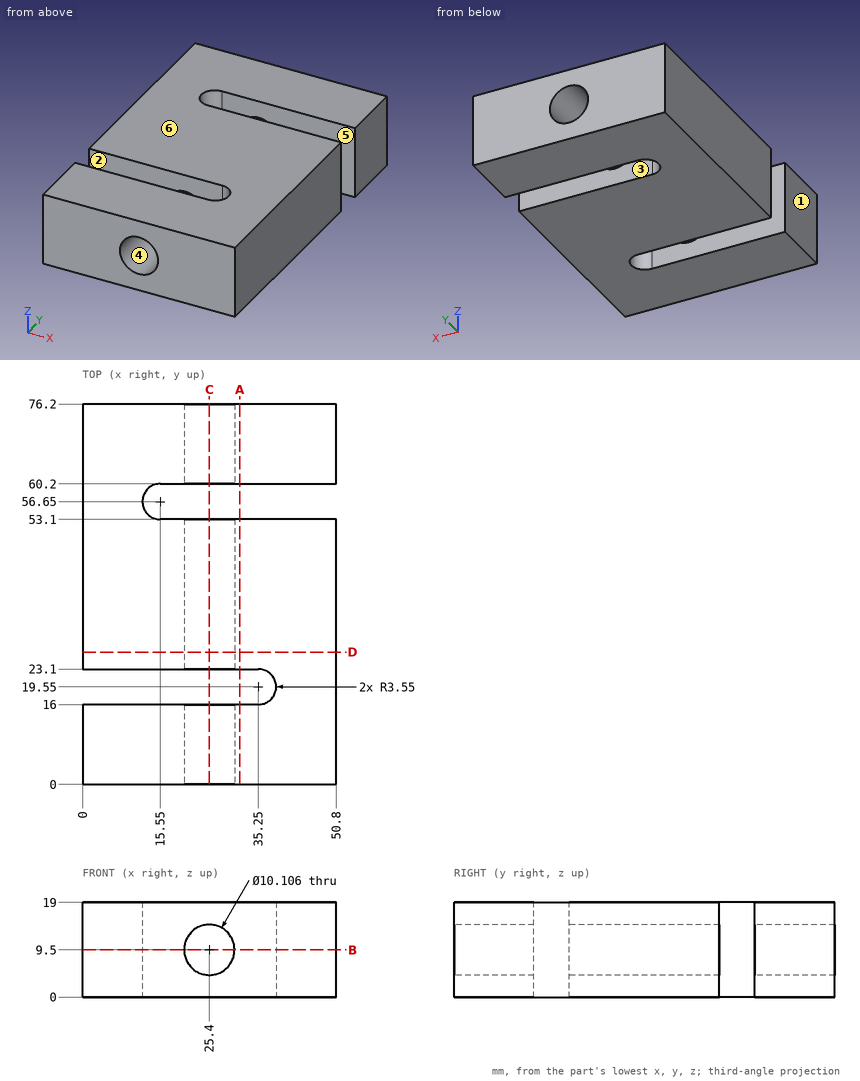
For this review, use the dimensioned drawing (mm, ordinates from the lowest corner) and the shaded views. A direction names the side the tool comes from. Round coordinates to 2 decimals unless told otherwise and drop trailing zeros. Loops run counter-clockwise (first coordinate to the right, second up) from the corner with the lowest first, then second, coordinate; pieces in that order, holes last. Notation, with made-up numbers: M -31.5,20.5 L -5.5,20.5 A25 cw -5.5,52.5 Z; hole C 51.25,-4.5 d9. An arc over 180 degrees is marked long. Answer as CSV lines item,"result".
1. We need section D-D (y = 26.5). Give the boundary of the cut face in (x, z), plus the area to 3 significant figures.
Outcome:
outline,"M 0,0 L 50.8,0 L 50.8,19 L 0,19 Z; hole C 25.4,9.5 d10.11"
area,"885 mm2"
2. We need section B-B (z = 9.5). Give the boundary of the cut face in (x, y).
Outcome:
outline,"M 0,0 L 20.35,0 L 20.35,16 L 0,16 Z; M 0,23.1 L 20.35,23.1 L 20.35,53.1 L 15.55,53.1 A3.55 cw 15.55,60.2 L 20.35,60.2 L 20.35,76.2 L 0,76.2 Z; M 30.45,0 L 50.8,0 L 50.8,53.1 L 30.45,53.1 L 30.45,23.1 L 35.25,23.1 A3.55 cw 35.25,16 L 30.45,16 Z; M 30.45,60.2 L 50.8,60.2 L 50.8,76.2 L 30.45,76.2 Z"
3. We need section A-A (x = 31.5). Give the boundary of the cut face in (y, z).
Outcome:
outline,"M 0,0 L 16,0 L 16,19 L 0,19 Z; M 23.1,0 L 53.1,0 L 53.1,19 L 23.1,19 Z; M 60.2,0 L 76.2,0 L 76.2,19 L 60.2,19 Z"
4. To check wall thickness, follow L1, parallel to Y at x = 16.5, z = 4.25; L2, parallel to Y at x = 7.5, z = 8.75; L3, parallel to Y at x = 43.5, z = 6.75. State the ranges of each line that lie inside material, in increasing order. Write a range as [from, to].
Outcome:
L1,"y = [0, 16], [23.1, 53.1], [60.2, 76.2]"
L2,"y = [0, 16], [23.1, 76.2]"
L3,"y = [0, 53.1], [60.2, 76.2]"
5. Draft analysis for pull direction Z (two halves, no side actions). For the marked faces 4, 5 and 6, state which applies: pulls with the +Z half, pulls with the -Z half, needs draft (parallel to the pull), parting line crosses it, or undercut.
Outcome:
face 4,"undercut"
face 5,"needs draft"
face 6,"pulls with the +Z half"
6. For the marked faces 1, 2 and 3, list the 3-axis set-ups (+Z, -Z, +X, -X, +Y, -Y) from which the entire face can be reached by the end or side of a thin tool; tool diameter is ignored.
Outcome:
face 1,"+Z, -Z, -X, +Y, -Y"
face 2,"+Z, -Z, -X"
face 3,"+Z, -Z, +X"
7. We need section C-C (x = 25.4). Give the boundary of the cut face in (y, z).
Outcome:
outline,"M 0,0 L 16,0 L 16,4.45 L 0,4.45 Z; M 0,14.55 L 16,14.55 L 16,19 L 0,19 Z; M 23.1,0 L 53.1,0 L 53.1,4.45 L 23.1,4.45 Z; M 23.1,14.55 L 53.1,14.55 L 53.1,19 L 23.1,19 Z; M 60.2,0 L 76.2,0 L 76.2,4.45 L 60.2,4.45 Z; M 60.2,14.55 L 76.2,14.55 L 76.2,19 L 60.2,19 Z"
